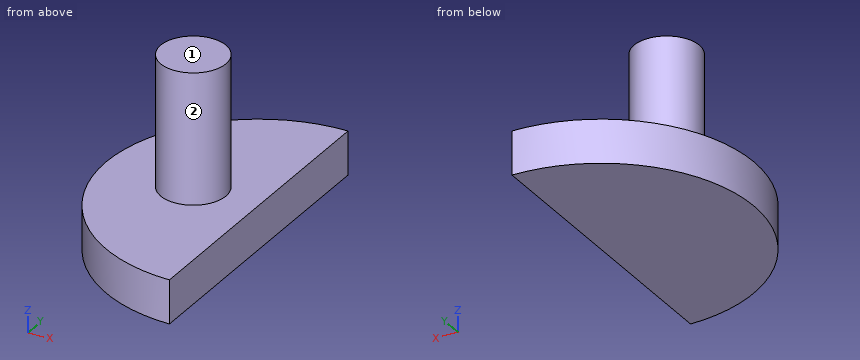
from build123d import *

# Parameters (mm, degrees)
F0_R     = 19.05
F1_DEPTH = 101.6
F2_DEPTH = 25.4
F3_DEPTH = 76.2


with BuildPart() as f1:
    # F0 (on Top) → F1 (new body)
    with BuildSketch(Plane.XY):
        with Locations((-38.1, 0)):
            Circle(F0_R)
    extrude(amount=F1_DEPTH)

    # F0 (on Top) → F2 (join)
    with BuildSketch(Plane.XY):
        with BuildLine():
            Line((0, -88.9), (0, 88.9))
            ThreePointArc((0, 88.9), (-88.9, 0), (0, -88.9))
        make_face()
        with Locations((-38.1, 0)):
            Circle(F0_R, mode=Mode.SUBTRACT)
    extrude(amount=F2_DEPTH)

    # F3 (cut): a face of the model
    f3_faces = [f1.faces().sort_by_distance(p)[0] for p in [
        (-38.1, 0, 101.6),
    ]]
    extrude(f3_faces, amount=F3_DEPTH, mode=Mode.SUBTRACT)


solid = f1.part
For this review, take the finished solid that the model builds, in its own axes (mm). Face numbers are marked on the shaded views. A direction names the side the tool comes from. Coordinates: 2 decimals unless noted, no trailing zeros. Write each loop counter-clockwise with the first axis right and the second up, starting at its lowest first coordinate (ties: lowest second). Pieces come first, ordered by that corner, then holes. Notation, with made-up numbers: (-8.75, 74) -> (42.25, 74) arc R32 ccw to (42.25, 111) -> close; hole circle Ø11 at (-30.75, 5.25). An arc over 180 degrees is marked (long way). Write each question's results on one line, items separated by ' | '. Start each with the question number.
1) Consider section D-D (x = -17). Write out the cut boundary in (y, z).
2) Consider section A-A (y = 0). Write out the cut boundary in (x, z).
3) Wall thickness on L1, parallel to Z at x = -24.5, y = 75.5; L2, parallel to Y at x = -21, z = 53; L3, parallel to X at y = -5.5, z = 15.5: over which ranges is each line inside the solid? List them lowest first. Write a range as [from, to].
4) Insertion check: pin 1 (3 mm diameter, centred on x = -72, y = -48, fed in from +Z). The pin has a flat end and moves straight along its axis. Give the tip position at first contact, or say it passes through.
5) Consider section C-C (z = 57). Write out the cut boundary in (x, y).
6) For the marked faces 1 and 2, list the 3-axis set-ups (+Z, -Z, +X, -X, +Y, -Y) from which the entire face can be reached by the end or side of a thin tool; tool diameter is ignored.
7) Consider section B-B (x = -45). Write out the cut boundary in (y, z).
Geometry says:
1) outline: (-87.26, 0) -> (87.26, 0) -> (87.26, 25.4) -> (-87.26, 25.4) -> close
2) outline: (-88.9, 0) -> (0, 0) -> (0, 25.4) -> (-19.05, 25.4) -> (-19.05, 101.6) -> (-57.15, 101.6) -> (-57.15, 25.4) -> (-88.9, 25.4) -> close
3) L1: [0, 25.4] | L2: [-8.4, 8.4] | L3: [-88.73, 0]
4) pin 1: z = 25.4
5) outline: circle Ø38.1 at (-38.1, 0)
6) face 1: +Z, +X, -X, +Y, -Y | face 2: +Z
7) outline: (-76.67, 0) -> (76.67, 0) -> (76.67, 25.4) -> (17.76, 25.4) -> (17.76, 101.6) -> (-17.76, 101.6) -> (-17.76, 25.4) -> (-76.67, 25.4) -> close
